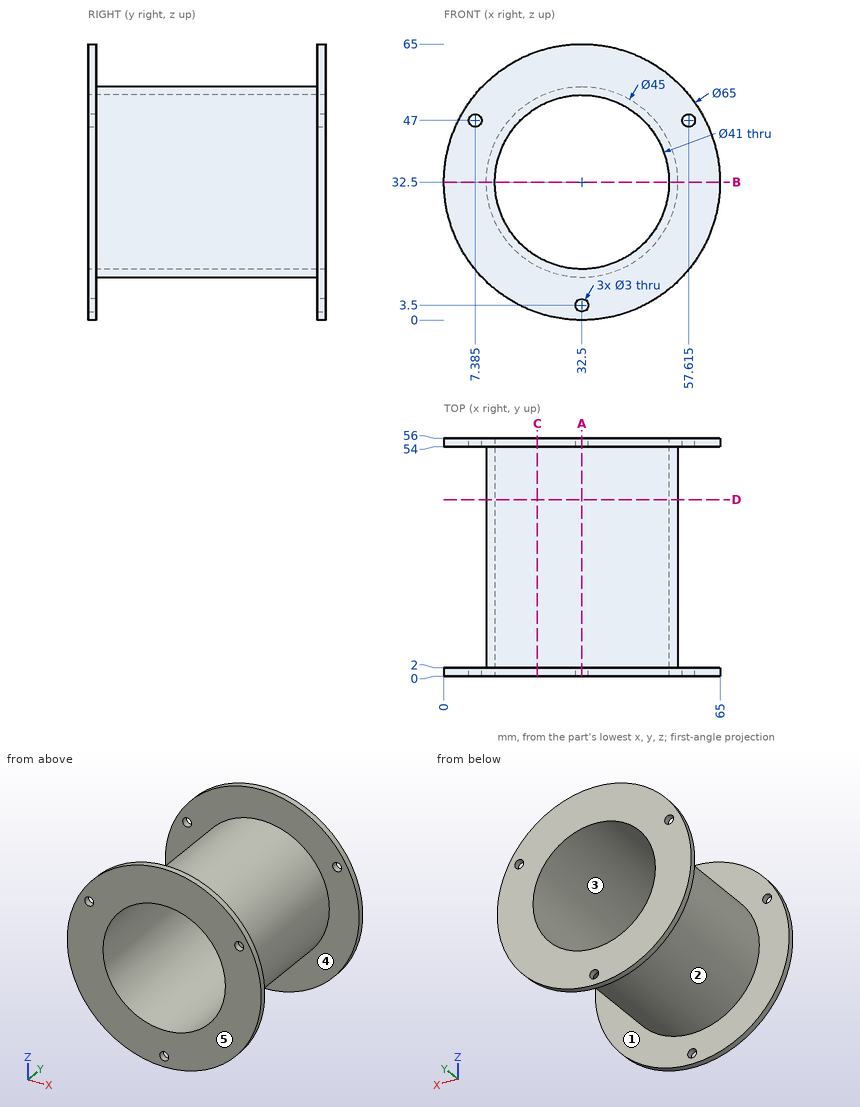
Job drawing, mm, ordinate dimensions from the low corner. One solid piece. A direction names the side the tool comes from. Round coordinates to 2 decimals unless told otherwise and drop trailing zeros. Loops run counter-clockwise (first coordinate to the right, second up) from the corner with the lowest first, then second, coordinate; pieces in that order, holes last. Notation, with made-up numbers: (35, -37) -> (49, -37) arc R10 ccw to (49, -27) -> close; hole circle Ø2 at (11, 31.5). An arc over 180 degrees is marked (long way). Use CSV: the item, a comma, the result in double quotes. Start each with the question number.
Q1. Which spindle directions (+Z, -Z, +X, -X, +Y, -Y) get a long thin tool onto all of the face, cutting with end or side? Do the marked faces 4 and 5. Say none if no direction does.
Q2. Flat gauge pins, fed straight in: pin 1 Ø1 at (y, z) = (14, 32) entering from +X; pin 2 Ø4 at (x, y) = (41, 13) entering from +Z; pin 3 Ø2.5 at (x, z) = (32.5, 3.5) entering from -Y; pin 4 Ø5 at (y, z) = (46.5, 24.5) entering from +X. Where does each tip first touch, or does it go through?
Q3. Saw through at C-C on x = 22. Give the cut face in (y, z).
Q4. Saw through at D-D on y = 41.5. Give the cut face in (x, z).
Q5. Drill centre lines: L1, parallel to Z at x = 32, y = 31 (1 decimal); L2, parallel to Y at x = 20, z = 54; L3, parallel to X at y = 1.4, z = 47 (1 decimal). Where is each one in solid material? Low to high.
Q6. Mould opens along X. For the marked faces 1, 2 and 3 say: +X half, -X half, draft (parallel to the pull), parting line (faces both ways), or undercut.
Q7. Saw through at A-A on x = 32.5. Give the cut face in (y, z).
Q8. Saw through at B-B on z = 32.5. Give the cut face in (x, y).
Solutions:
1,face 4,"none"
1,face 5,"+Z, -Z, +X, -X, -Y"
2,pin 1,"stops at x = 55"
2,pin 2,"stops at z = 54.04"
2,pin 3,"passes through"
2,pin 4,"stops at x = 54.32"
3,outline,"(0, 1.74) -> (2, 1.74) -> (2, 12.6) -> (54, 12.6) -> (54, 1.74) -> (56, 1.74) -> (56, 14.89) -> (0, 14.89) -> close; (0, 50.11) -> (56, 50.11) -> (56, 63.26) -> (54, 63.26) -> (54, 52.4) -> (2, 52.4) -> (2, 63.26) -> (0, 63.26) -> close"
4,outline,"circle Ø45 at (32.5, 32.5); hole circle Ø41 at (32.5, 32.5)"
5,L1,"z = 10 to 12, 53 to 55"
5,L2,"y = 0 to 2, 54 to 56"
5,L3,"x = 3.4 to 5.9, 8.9 to 18, 47 to 56.1, 59.1 to 61.6"
6,face 1,"draft"
6,face 2,"parting line"
6,face 3,"undercut"
7,outline,"(0, 0) -> (2, 0) -> (2, 2) -> (0, 2) -> close; (0, 5) -> (2, 5) -> (2, 10) -> (54, 10) -> (54, 5) -> (56, 5) -> (56, 12) -> (0, 12) -> close; (0, 53) -> (56, 53) -> (56, 65) -> (54, 65) -> (54, 55) -> (2, 55) -> (2, 65) -> (0, 65) -> close; (54, 0) -> (56, 0) -> (56, 2) -> (54, 2) -> close"
8,outline,"(0, 0) -> (12, 0) -> (12, 56) -> (0, 56) -> (0, 54) -> (10, 54) -> (10, 2) -> (0, 2) -> close; (53, 0) -> (65, 0) -> (65, 2) -> (55, 2) -> (55, 54) -> (65, 54) -> (65, 56) -> (53, 56) -> close"
